Verification items for the finished model (mm, model axes). A direction names the side the tool comes from. Round coordinates to 2 decimals unless told otherwise and drop trailing zeros. Write each loop counter-clockwise with the first axis right and the second up, starting at its lowest first coordinate (ties: lowest second). Pieces come first, ordered by that corner, then holes. Notation, with made-up numbers: M 69,47.5 L 114,47.5 A13 cw 114,69.5 Z; hole C 51,61 d1. An arc over 180 degrees is marked long. One line per item, written item: value. Start each with the question number.
Item 1: Section check A-A, the plane x = 73. Record the cut outline in (y, z), then the cut area to 3 significant figures.
Item 2: Section check C-C, the plane z = 0.65. Record the cut outline in (x, y).
Item 3: Draft check along Y on faces 3 (the face through (72, 19, 1)), 4 (the face through (67, 0, 1)), 5 (the face through (67.285, -18.699, 0.986)), 6 (the face through (72, 11, 1)). Enter one of: +Y half, -Y half, draft (parallel to the pull), parting line (faces both ways), or undercut.
Item 4: Tool access check on faces 1 (the face through (69.5, 13, 1)), 2 (the face through (77.715, 18.699, 0.986)). Record the directions out of +Z, -Z, +X, -X, +Y, -Y that give a thin tool (end or side, any length) a straight path to the whole face; none if there is none.
Item 5: Thickness scan on probe 1 along X at (y, z) = (12, 1.7); probe 2 along X at (y, z) = (-5, 1.3); probe 3 along Y at (x, z) = (71.5, 1.15). Record the ranges inside material, lowest first. Write a range as from..to.
Item 6: Section check D-D, the plane x = 71.5. Record the cut outline in (y, z).
Item 7: Section check B-B, the plane y = 5. Record the cut outline in (x, z).
from build123d import *

# Parameters (mm, degrees)
SKETCH324_R      = 1.5
EXTRUDE192_DEPTH = 10
SKETCH321_W      = 6
SKETCH321_H      = 4
EXTRUDE189_DEPTH = 3
SKETCH319_R      = 1
EXTRUDE187_DEPTH = 5
EXTRUDE188_DEPTH = 2


with BuildPart() as extrude192:
    # Sketch324 → Extrude192 (new body)
    with BuildSketch(Plane.XY.offset(-2)):
        with Locations((72.5, -12.5)):
            Circle(SKETCH324_R)
    extrude(amount=EXTRUDE192_DEPTH)


with BuildPart() as extrude189:
    # Sketch321 → Extrude189 (new body)
    with BuildSketch(Plane.XY.offset(3)):
        with Locations((72.5, 13)):
            Rectangle(SKETCH321_W, SKETCH321_H)
    extrude(amount=EXTRUDE189_DEPTH)


with BuildPart() as extrude187:
    # Sketch319 → Extrude187 (new body)
    with BuildSketch(Plane.XY.offset(3)):
        with Locations((71.5, 5)):
            Circle(SKETCH319_R)
        with Locations((71.5, -5)):
            Circle(SKETCH319_R)
    extrude(amount=EXTRUDE187_DEPTH)


with BuildPart() as obj1:
    # Sketch318 → Extrude188 (new body)
    with BuildSketch(Plane.XY.offset(3)):
        with BuildLine():
            Line((67, -18), (67, 18))
            ThreePointArc((68, 19), (67.292893, 18.707107), (67, 18))
            Line((68, 19), (77, 19))
            ThreePointArc((78, 18), (77.707107, 18.707107), (77, 19))
            Line((78, 18), (78, -18))
            ThreePointArc((77, -19), (77.707107, -18.707107), (78, -18))
            Line((68, -19), (77, -19))
            ThreePointArc((67, -18), (67.292893, -18.707107), (68, -19))
        make_face()
    extrude(amount=EXTRUDE188_DEPTH)

    # Cut098: cut Extrude187
    add(extrude187.part, mode=Mode.SUBTRACT)

    # Cut099: cut Extrude189
    add(extrude189.part, mode=Mode.SUBTRACT)


with BuildPart() as obj1_1:
    # Cut099 placement: moved
    add(obj1.part.moved(Location((0, 0, -3))))

    # Cut102: cut Extrude192
    add(extrude192.part, mode=Mode.SUBTRACT)


solid = obj1_1.part
Response values:
1. outline: M -19,0 L -13.91,0 L -13.91,2 L -19,2 Z; M -11.09,0 L 11,0 L 11,2 L -11.09,2 Z; M 15,0 L 19,0 L 19,2 L 15,2 Z
1. area: 62.3 mm2
2. outline: M 67,-18 A1 ccw 68,-19 L 77,-19 A1 ccw 78,-18 L 78,18 A1 ccw 77,19 L 68,19 A1 ccw 67,18 Z; hole M 69.5,11 L 75.5,11 L 75.5,15 L 69.5,15 Z; hole C 71.5,-5 d2; hole C 71.5,5 d2; hole C 72.5,-12.5 d3
3. face 3: +Y half
3. face 4: draft
3. face 5: -Y half
3. face 6: undercut
4. face 1: +Z, -Z
4. face 2: +Z, -Z, +X, +Y
5. probe 1: x = 67..69.5, 75.5..78
5. probe 2: x = 67..70.5, 72.5..78
5. probe 3: y = -19..-13.62, -11.38..-6, -4..4, 6..11, 15..19
6. outline: M -19,0 L -13.62,0 L -13.62,2 L -19,2 Z; M -11.38,0 L -6,0 L -6,2 L -11.38,2 Z; M -4,0 L 4,0 L 4,2 L -4,2 Z; M 6,0 L 11,0 L 11,2 L 6,2 Z; M 15,0 L 19,0 L 19,2 L 15,2 Z
7. outline: M 67,0 L 70.5,0 L 70.5,2 L 67,2 Z; M 72.5,0 L 78,0 L 78,2 L 72.5,2 Z
